```python
from build123d import *

# Parameters (mm, degrees)
SKETCH_1_W          = 68
SKETCH_1_H          = 44
EXTRUDE_1_DEPTH     = 2
FILLET_1_R          = 5.5
CUT_EXTRUDE_1_DEPTH = 1
CUT_EXTRUDE_2_DEPTH = 1
CUT_EXTRUDE_3_REACH = 65.352
SKETCH_5_R          = 1.325
CUT_EXTRUDE_5_DEPTH = 64.328343814
SKETCH_6_R          = 2.6
CUT_EXTRUDE_6_DEPTH = 1.5
CHAMFER_2_SIZE      = 1.4


with BuildPart() as part:
    # 草图1 → 凸台-拉伸1 (new body)
    with BuildSketch(Plane(origin=(0, 0, 0), x_dir=(1, 0, 0), z_dir=(0, 1, 0))):
        with Locations((23.975845411, -3.461352657)):
            Rectangle(SKETCH_1_W, SKETCH_1_H)
    extrude(amount=EXTRUDE_1_DEPTH)

    # 圆角1
    fillet_1_edges = [part.edges().sort_by_distance(p)[0] for p in [
        (-10.024154589, 1, -18.538647343),
        (57.975845411, 1, -18.538647343),
        (57.975845411, 1, 25.461352657),
        (-10.024154589, 1, 25.461352657),
    ]]
    fillet(fillet_1_edges, radius=FILLET_1_R)

    # 草图3 → 切除-拉伸1 (cut)
    with BuildSketch(Plane(origin=(0, 2, 0), x_dir=(1, 0, 0), z_dir=(0, 1, 0))):
        with BuildLine():
            Line((3.975845411, 6.038647343), (43.975845411, 6.038647343))
            ThreePointArc((43.975845411, 6.038647343), (47.157825926, 4.720627858), (48.475845411, 1.538647343))
            Line((48.475845411, 1.538647343), (48.475845411, -20.961352657))
            ThreePointArc((48.475845411, -20.961352657), (47.157825926, -24.143333172), (43.975845411, -25.461352657))
            Line((43.975845411, -25.461352657), (3.975845411, -25.461352657))
            ThreePointArc((3.975845411, -25.461352657), (0.793864895, -24.143333172), (-0.524154589, -20.961352657))
            Line((-0.524154589, -20.961352657), (-0.524154589, 1.538647343))
            ThreePointArc((-0.524154589, 1.538647343), (0.793864895, 4.720627858), (3.975845411, 6.038647343))
        make_face()
    extrude(amount=-CUT_EXTRUDE_1_DEPTH, mode=Mode.SUBTRACT)

    # 草图4 → 切除-拉伸2 (cut)
    with BuildSketch(Plane(origin=(0, 1, 0), x_dir=(1, 0, 0), z_dir=(0, 1, 0))):
        with BuildLine():
            Line((43.475845411, -24.461352657), (16.475845411, -24.461352657))
            ThreePointArc((16.475845411, -24.461352657), (14.000971676, -23.436226391), (12.975845411, -20.961352657))
            Line((12.975845411, -20.961352657), (12.975845411, 1.338647343))
            ThreePointArc((12.975845411, 1.338647343), (14.000971676, 3.813521077), (16.475845411, 4.838647343))
            Line((16.475845411, 4.838647343), (43.475845411, 4.838647343))
            ThreePointArc((43.475845411, 4.838647343), (45.950719145, 3.813521077), (46.975845411, 1.338647343))
            Line((46.975845411, 1.338647343), (46.975845411, -20.961352657))
            ThreePointArc((46.975845411, -20.961352657), (45.950719145, -23.436226391), (43.475845411, -24.461352657))
        make_face()
    extrude(amount=-CUT_EXTRUDE_2_DEPTH, mode=Mode.SUBTRACT)

    # 草图5 → 切除-拉伸3 (cut, up to next)
    with BuildSketch(Plane(origin=(0, 2, 0), x_dir=(1, 0, 0), z_dir=(0, 1, 0)), mode=Mode.PRIVATE) as cut_extrude_3_sk1:
        with Locations(Location((53.000845411, -21.286352657, 0), (0, 0, 270))):
            Circle(SKETCH_5_R)
    cut_extrude_3_tool1 = extrude(cut_extrude_3_sk1.sketch, amount=-CUT_EXTRUDE_3_REACH, mode=Mode.PRIVATE) & part.part
    # 草图5 → 切除-拉伸3 (cut, up to next)
    with BuildSketch(Plane(origin=(0, 2, 0), x_dir=(1, 0, 0), z_dir=(0, 1, 0)), mode=Mode.PRIVATE) as cut_extrude_3_sk2:
        with Locations(Location((53.000845411, 1.763647343, 0), (0, 0, 270))):
            Circle(SKETCH_5_R)
    cut_extrude_3_tool2 = extrude(cut_extrude_3_sk2.sketch, amount=-CUT_EXTRUDE_3_REACH, mode=Mode.PRIVATE) & part.part
    # 草图5 → 切除-拉伸3 (cut, up to next)
    with BuildSketch(Plane(origin=(0, 2, 0), x_dir=(1, 0, 0), z_dir=(0, 1, 0)), mode=Mode.PRIVATE) as cut_extrude_3_sk3:
        with Locations(Location((-5.049154589, 1.763647343, 0), (0, 0, 270))):
            Circle(SKETCH_5_R)
    cut_extrude_3_tool3 = extrude(cut_extrude_3_sk3.sketch, amount=-CUT_EXTRUDE_3_REACH, mode=Mode.PRIVATE) & part.part
    # 草图5 → 切除-拉伸3 (cut, up to next)
    with BuildSketch(Plane(origin=(0, 2, 0), x_dir=(1, 0, 0), z_dir=(0, 1, 0)), mode=Mode.PRIVATE) as cut_extrude_3_sk4:
        with Locations(Location((-5.049154589, -21.286352657, 0), (0, 0, 270))):
            Circle(SKETCH_5_R)
    cut_extrude_3_tool4 = extrude(cut_extrude_3_sk4.sketch, amount=-CUT_EXTRUDE_3_REACH, mode=Mode.PRIVATE) & part.part
    add(cut_extrude_3_tool1.solids().sort_by_distance((53.000845, 2, 21.286353))[0], mode=Mode.SUBTRACT)
    add(cut_extrude_3_tool2.solids().sort_by_distance((53.000845, 2, -1.763647))[0], mode=Mode.SUBTRACT)
    add(cut_extrude_3_tool3.solids().sort_by_distance((-5.049155, 2, -1.763647))[0], mode=Mode.SUBTRACT)
    add(cut_extrude_3_tool4.solids().sort_by_distance((-5.049155, 2, 21.286353))[0], mode=Mode.SUBTRACT)

    # 草图7 → 切除-拉伸5 (cut, through all)
    with BuildSketch(Plane(origin=(0, 1, 0), x_dir=(1, 0, 0), z_dir=(0, 1, 0))):
        with BuildLine():
            Line((7.975835944, -6.705199166), (7.994321526, -12.713332009))
            ThreePointArc((7.994321526, -12.713332009), (6.000484483, -14.719476033), (3.994340459, -12.72563899))
            Line((3.994340459, -12.72563899), (3.975854877, -6.717506148))
            ThreePointArc((3.975854877, -6.717506148), (5.96969192, -4.711362123), (7.975835944, -6.705199166))
        make_face()
    extrude(amount=-CUT_EXTRUDE_5_DEPTH, mode=Mode.SUBTRACT)

    # 草图6 → 切除-拉伸6 (cut)
    with BuildSketch(Plane(origin=(0, 2, 0), x_dir=(1, 0, 0), z_dir=(0, 1, 0))):
        with Locations(Location((-5.049154589, 1.763647343, 0), (0, 0, 270))):
            Circle(SKETCH_6_R)
        with Locations(Location((-5.049154589, -21.286352657, 0), (0, 0, 270))):
            Circle(SKETCH_6_R)
        with Locations(Location((53.000845411, 1.763647343, 0), (0, 0, 270))):
            Circle(SKETCH_6_R)
        with Locations(Location((53.000845411, -21.286352657, 0), (0, 0, 270))):
            Circle(SKETCH_6_R)
    extrude(amount=-CUT_EXTRUDE_6_DEPTH, mode=Mode.SUBTRACT)

    # 倒角2
    # the kernel refuses this chamfer: 1.4 mm, written as the material it adds along each edge
    with BuildSketch(Plane(origin=(53.000845411, 0.5, 21.286352657), x_dir=(0, 0, 1), z_dir=(-1, 0, 0))) as chamfer_2_piece_1_section:
        Polygon((2.6, CHAMFER_2_SIZE), (2.6 - CHAMFER_2_SIZE, 0), (2.6, 0), align=None)
    chamfer_2_piece_1 = revolve(axis=Axis((53.000845411, 0.5, 21.286352657), (0, 1, 0)), mode=Mode.PRIVATE)
    chamfer_2_piece_1 = chamfer_2_piece_1 - Plane(origin=(53.000845411, 1.265114472, 21.286352657), x_dir=(0, 0, 1), z_dir=(0, 1, 0)) * Cylinder(1.325, 11, mode=Mode.PRIVATE)
    add(chamfer_2_piece_1)
    with BuildSketch(Plane(origin=(-5.049154589, 0.5, 21.286352657), x_dir=(0, 0, 1), z_dir=(-1, 0, 0))) as chamfer_2_piece_2_section:
        Polygon((2.6, CHAMFER_2_SIZE), (2.6 - CHAMFER_2_SIZE, 0), (2.6, 0), align=None)
    chamfer_2_piece_2 = revolve(axis=Axis((-5.049154589, 0.5, 21.286352657), (0, 1, 0)), mode=Mode.PRIVATE)
    chamfer_2_piece_2 = chamfer_2_piece_2 - Plane(origin=(-5.049154589, 1.265114472, 21.286352657), x_dir=(0, 0, 1), z_dir=(0, 1, 0)) * Cylinder(1.325, 11, mode=Mode.PRIVATE)
    add(chamfer_2_piece_2)
    with BuildSketch(Plane(origin=(-5.049154589, 0.5, -1.763647343), x_dir=(0, 0, 1), z_dir=(-1, 0, 0))) as chamfer_2_piece_3_section:
        Polygon((2.6, CHAMFER_2_SIZE), (2.6 - CHAMFER_2_SIZE, 0), (2.6, 0), align=None)
    chamfer_2_piece_3 = revolve(axis=Axis((-5.049154589, 0.5, -1.763647343), (0, 1, 0)), mode=Mode.PRIVATE)
    chamfer_2_piece_3 = chamfer_2_piece_3 - Plane(origin=(-5.049154589, 1.265114472, -1.763647343), x_dir=(0, 0, 1), z_dir=(0, 1, 0)) * Cylinder(1.325, 11, mode=Mode.PRIVATE)
    add(chamfer_2_piece_3)
    with BuildSketch(Plane(origin=(53.000845411, 0.5, -1.763647343), x_dir=(0, 0, 1), z_dir=(-1, 0, 0))) as chamfer_2_piece_4_section:
        Polygon((2.6, CHAMFER_2_SIZE), (2.6 - CHAMFER_2_SIZE, 0), (2.6, 0), align=None)
    chamfer_2_piece_4 = revolve(axis=Axis((53.000845411, 0.5, -1.763647343), (0, 1, 0)), mode=Mode.PRIVATE)
    chamfer_2_piece_4 = chamfer_2_piece_4 - Plane(origin=(53.000845411, 1.265114472, -1.763647343), x_dir=(0, 0, 1), z_dir=(0, 1, 0)) * Cylinder(1.325, 11, mode=Mode.PRIVATE)
    add(chamfer_2_piece_4)


solid = part.part
```
Check sheet for the modelled part. Datum: model origin and axes. Units: mm. A direction names the side the tool comes from. Round coordinates to 2 decimals unless told otherwise and drop trailing zeros. Write each loop counter-clockwise with the first axis right and the second up, starting at its lowest first coordinate (ties: lowest second). Pieces come first, ordered by that corner, then holes. Notation, with made-up numbers: (19.5, 75) -> (23.5, 75) arc R19 ccw to (23.5, 81) -> close; hole circle Ø9 at (-20, -28.75). An arc over 180 degrees is marked (long way). One line per question, with ' | ' between items. Start each with the question number.
1. Scan lines: line 1 along X through (y, z) = (0.3, 11); line 2 along X through (y, z) = (0.35, 18.5); line 3 along Z through (x, y) = (40, 0.85). Record each from-to range of solid material in increasing order. Write a range as from..to.
2. Sectioned sample at C-C, the plane z = 11. Record the cut outline in (x, y).
3. Sectioned sample at D-D, the plane y = 1.5. Record the cut outline in (x, z).
4. Set-up check for faces 5 (the face through (56.41, 1.01, -16.88)), 6 (the face through (0.83, 1.51, 24.18)), 7 (the face through (14.028, 0.507, 23.463)): record each of +Z, -Z, +X, -X, +Y, -Y from which the full face is reachable in a straight line by a thin tool's end or side.
5. Depth check by flat-ended pin: pin 1 (4 mm diameter, centred on x = 53, z = 21.29, fed in from +Y); pin 2 (3.5 mm diameter, centred on x = -5.05, z = -1.76, fed in from -Y); pin 3 (0.5 mm diameter, centred on x = 24.5, y = 1.5, fed in from +Z). Enter the tip coordinate at first touch or a pass-through.
6. Release check for a two-part mould opening along Z. For faces 1 (the face through (45.923, 0.507, -3.841)), 2 (the face through (57.976, 1, 4)), 3 (the face through (23.6, 0.8, 25.461)), 4 (the face through (24, 1, -18.539)) record: +Z half, -Z half, draft (parallel to the pull), parting line (faces both ways), or undercut.
7. Sectioned sample at B-B, the plane x = 23. Record the cut outline in (y, z).
8. Sectioned sample at A-A, the plane z = 17.5. Record the cut outline in (x, y).
Taken from the geometry:
1) line 1: x = -10.02..3.99, 7.99..12.98, 46.98..57.98 | line 2: x = -10.02..12.98, 46.98..57.98 | line 3: z = -18.54..-4.84, 24.46..25.46
2) outline: (-10.02, 0) -> (3.99, 0) -> (3.99, 1) -> (-0.52, 1) -> (-0.52, 2) -> (-10.02, 2) -> close; (7.99, 0) -> (12.98, 0) -> (12.98, 1) -> (7.99, 1) -> close; (46.98, 0) -> (57.98, 0) -> (57.98, 2) -> (48.48, 2) -> (48.48, 1) -> (46.98, 1) -> close
3) outline: (-10.02, -13.04) arc R5.5 ccw to (-4.52, -18.54) -> (52.48, -18.54) arc R5.5 ccw to (57.98, -13.04) -> (57.98, 19.96) arc R5.5 ccw to (52.48, 25.46) -> (43.98, 25.46) arc R4.5 cw to (48.48, 20.96) -> (48.48, -1.54) arc R4.5 cw to (43.98, -6.04) -> (3.98, -6.04) arc R4.5 cw to (-0.52, -1.54) -> (-0.52, 20.96) arc R4.5 cw to (3.98, 25.46) -> (-4.52, 25.46) arc R5.5 ccw to (-10.02, 19.96) -> close; hole circle Ø4.4 at (-5.05, -1.76); hole circle Ø4.4 at (-5.05, 21.29); hole circle Ø4.4 at (53, -1.76); hole circle Ø4.4 at (53, 21.29)
4) face 5: -Z, +X, +Y, -Y | face 6: +Y | face 7: +Y, -Y
5) pin 1: stops at y = 1.3 | pin 2: stops at y = 0 | pin 3: stops at z = -6.04
6) face 1: undercut | face 2: draft | face 3: +Z half | face 4: -Z half
7) outline: (0, -18.54) -> (2, -18.54) -> (2, -6.04) -> (1, -6.04) -> (1, -4.84) -> (0, -4.84) -> close; (0, 24.46) -> (1, 24.46) -> (1, 25.46) -> (0, 25.46) -> close
8) outline: (-10.02, 0) -> (12.98, 0) -> (12.98, 1) -> (-0.52, 1) -> (-0.52, 2) -> (-10.02, 2) -> close; (46.98, 0) -> (57.98, 0) -> (57.98, 2) -> (48.48, 2) -> (48.48, 1) -> (46.98, 1) -> close
